```python
from build123d import *

# Parameters (mm, degrees)
SKETCH1_R           = 2.5527
SKETCH1_R_2         = 19.685
SKETCH1_W           = 12.7
SKETCH1_H           = 12.7
BOSS_EXTRUDE1_DEPTH = 14.605
CUT_EXTRUDE1_DEPTH  = 6.35
BOSS_EXTRUDE2_START = -5.842
SKETCH3_R           = 19.685
SKETCH3_R_2         = 14.2875
BOSS_EXTRUDE2_DEPTH = 5.842
SKETCH4_R           = 2.5527
CUT_EXTRUDE2_DEPTH  = 93.738266239
CUT_EXTRUDE3_DEPTH  = 6.35
CUT_EXTRUDE4_START  = -7.62
SKETCH8_R           = 2.5527
CUT_EXTRUDE4_DEPTH  = 7.62
FILLET1_R           = 3.81
FILLET3_R           = 0.0635
FILLET4_START       = 6.985
FILLET4_DEPTH       = 9.015
CHAMFER1_SIZE       = 3.81
FILLET5_R           = 2.54


with BuildPart() as part:
    # Sketch1 → Boss-Extrude1 (new body)
    # profile 1 of 3: a face of its own
    with BuildSketch(Plane.XY):
        Polygon((0, 63.5), (0, 0), (50.8, 0), (50.8, 63.5), (38.1, 63.5), (12.7, 63.5), align=None)
        with Locations(Location((6.35, 6.35, 0), (0, 0, 180))):
            Circle(SKETCH1_R, mode=Mode.SUBTRACT)
        with Locations(Location((5.668864874, 22.104928677, 0), (0, 0, 180))):
            Circle(SKETCH1_R, mode=Mode.SUBTRACT)
        with Locations(Location((44.45, 6.35, 0), (0, 0, 180))):
            Circle(SKETCH1_R, mode=Mode.SUBTRACT)
        with Locations(Location((44.45, 19.05, 0), (0, 0, 180))):
            Circle(SKETCH1_R, mode=Mode.SUBTRACT)
        with Locations(Location((25.4, 38.1, 0), (0, 0, 180))):
            Circle(SKETCH1_R_2, mode=Mode.SUBTRACT)
        with Locations(Location((45.131135126, 54.095071323, 0), (0, 0, 180))):
            Circle(SKETCH1_R, mode=Mode.SUBTRACT)
    # profile 2 of 3: a face of its own
    with BuildSketch(Plane.XY):
        with Locations((6.35, 69.85)):
            Rectangle(SKETCH1_W, SKETCH1_H)
        with Locations(Location((6.35, 69.85, 0), (0, 0, 180))):
            Circle(SKETCH1_R, mode=Mode.SUBTRACT)
    # profile 3 of 3: a face of its own
    with BuildSketch(Plane.XY):
        with Locations((44.45, 69.85)):
            Rectangle(SKETCH1_W, SKETCH1_H)
        with Locations(Location((44.45, 67.945, 0), (0, 0, 180))):
            Circle(SKETCH1_R, mode=Mode.SUBTRACT)
    extrude(amount=BOSS_EXTRUDE1_DEPTH)

    # Sketch2 → Cut-Extrude1 (cut)
    with BuildSketch(Plane(origin=(0, 0, 0), x_dir=(-1, 0, 0), z_dir=(0, 0, -1))):
        Polygon((-41.45488381, 58.476257037), (-47.087227595, 59.469391211), (-50.763478911, 55.088205497), (-48.807386443, 49.713885609), (-43.175042658, 48.720751435), (-39.498791341, 53.101937149), align=None)
        Polygon((-1.992613557, 26.486114391), (-7.624957342, 27.479248565), (-11.301208659, 23.098062851), (-9.34511619, 17.723742963), (-3.712772405, 16.730608789), (-0.036521089, 21.111794503), align=None)
        Polygon((-41.590384117, 11.303), (-47.309615883, 11.303), (-50.169231767, 6.35), (-47.309615883, 1.397), (-41.590384117, 1.397), (-38.730768233, 6.35), align=None)
        Polygon((-44.45, 73.664231767), (-49.403, 70.804615883), (-49.403, 65.085384117), (-44.45, 62.225768233), (-39.497, 65.085384117), (-39.497, 70.804615883), align=None)
    extrude(amount=-CUT_EXTRUDE1_DEPTH, mode=Mode.SUBTRACT)

    # Sketch3 → Boss-Extrude2 (add)
    with BuildSketch(Plane.XY.offset(14.605).offset(BOSS_EXTRUDE2_START)):
        with Locations(Location((25.4, 38.1, 0), (0, 0, 180))):
            Circle(SKETCH3_R)
        with Locations((25.4, 38.1)):
            Circle(SKETCH3_R_2, mode=Mode.SUBTRACT)
    extrude(amount=BOSS_EXTRUDE2_DEPTH)

    # Sketch4 → Cut-Extrude2 (cut, through all)
    with BuildSketch(Plane.XY.offset(14.605)):
        with Locations((6.35, 54.61)):
            Circle(SKETCH4_R)
    extrude(amount=-CUT_EXTRUDE2_DEPTH, mode=Mode.SUBTRACT)

    # Sketch5 → Cut-Extrude3 (cut)
    with BuildSketch(Plane(origin=(0, 0, 0), x_dir=(-1, 0, 0), z_dir=(0, 0, -1))):
        Polygon((-2.673748684, 50.228814286), (-0.717656215, 55.603134174), (-4.393907531, 59.984319888), (-10.026251316, 58.991185714), (-11.982343785, 53.616865826), (-8.306092469, 49.235680112), align=None)
    extrude(amount=-CUT_EXTRUDE3_DEPTH, mode=Mode.SUBTRACT)

    # Sketch8 → Cut-Extrude4 (cut)
    # profile 1 of 3: a face of its own
    with BuildSketch(Plane.XY.offset(14.605).offset(CUT_EXTRUDE4_START)):
        with BuildLine():
            Line((0, 76.2), (0, 69.85))
            ThreePointArc((0, 69.85), (6.35, 63.5), (12.7, 69.85))
            Line((12.7, 69.85), (12.7, 76.2))
            Line((12.7, 76.2), (0, 76.2))
        make_face()
        with Locations(Location((6.35, 69.85, 0), (0, 0, 180))):
            Circle(SKETCH8_R, mode=Mode.SUBTRACT)
    # profile 2 of 3: a face of its own
    with BuildSketch(Plane.XY.offset(14.605).offset(CUT_EXTRUDE4_START)):
        with BuildLine():
            Line((50.8, 25.4), (44.45, 25.4))
            ThreePointArc((44.45, 25.4), (38.1, 19.05), (44.45, 12.7))
            Line((44.45, 12.7), (50.8, 12.7))
            Line((50.8, 12.7), (50.8, 25.4))
        make_face()
        with Locations(Location((44.45, 19.05, 0), (0, 0, 180))):
            Circle(SKETCH8_R, mode=Mode.SUBTRACT)
    # profile 3 of 3: a face of its own
    with BuildSketch(Plane.XY.offset(14.605).offset(CUT_EXTRUDE4_START)):
        with BuildLine():
            Line((0, 0), (6.35, 0))
            ThreePointArc((6.35, 0), (10.840128061, 10.840128061), (0, 6.35))
            Line((0, 6.35), (0, 0))
        make_face()
        with Locations(Location((6.35, 6.35, 0), (0, 0, 180))):
            Circle(SKETCH8_R, mode=Mode.SUBTRACT)
    extrude(amount=CUT_EXTRUDE4_DEPTH, mode=Mode.SUBTRACT)

    # Fillet1
    fillet1_edges = [part.edges().sort_by_distance(p)[0] for p in [
        (0, 0, 3.4925),
        (0, 76.2, 3.4925),
        (12.7, 76.2, 3.4925),
        (12.7, 63.5, 7.3025),
        (38.1, 63.5, 7.3025),
        (38.1, 76.2, 7.3025),
        (50.8, 76.2, 7.3025),
        (50.8, 0, 7.3025),
    ]]
    fillet(fillet1_edges, radius=FILLET1_R)

    # Fillet3
    fillet3_edges = [part.edges().sort_by_distance(p)[0] for p in [
        (45.085, 38.1, 8.763),
    ]]
    fillet(fillet3_edges, radius=FILLET3_R)

    # Fillet4: read off the stored shape, not the designer's step
    # Fillet4 outline → Fillet4 (cut)
    with BuildSketch(Plane.XY.offset(FILLET4_START)):
        with BuildLine():
            ThreePointArc((14.382185257, 0), (12.23549345, 1.182312891), (12.087275183, 3.628571429))
            ThreePointArc((12.087275183, 3.628571429), (9.744217773, 0.983270482), (6.35, 0))
            Line((6.35, 0), (14.382185257, 0))
        make_face()
        with BuildLine():
            ThreePointArc((3.628571429, 12.087275183), (1.182312891, 12.23549345), (0, 14.382185257))
            Line((0, 14.382185257), (0, 6.35))
            ThreePointArc((0, 6.35), (0.983270482, 9.744217773), (3.628571429, 12.087275183))
        make_face()
        with BuildLine():
            ThreePointArc((0, 61.817814743), (1.182312891, 63.96450655), (3.628571429, 64.112724817))
            ThreePointArc((3.628571429, 64.112724817), (0.983270483, 66.455782228), (0, 69.85))
            Line((0, 69.85), (0, 61.817814743))
        make_face()
        with BuildLine():
            ThreePointArc((12.7, 69.85), (12.076615103, 67.106210748), (10.328856864, 64.901141742))
            ThreePointArc((10.328856864, 64.901141742), (12.086184936, 65.456182276), (13.756239766, 64.676959064))
            ThreePointArc((13.756239766, 64.676959064), (12.973905651, 65.891501938), (12.7, 67.31))
            Line((12.7, 67.31), (12.7, 69.85))
        make_face()
    extrude(amount=FILLET4_DEPTH, mode=Mode.SUBTRACT)

    # Chamfer1
    # the kernel refuses this chamfer: 3.81 mm, written as the material it takes off along each edge
    with BuildSketch(Plane(origin=(60.598112184, 25.4, 14.605), x_dir=(0, 1, 0), z_dir=(-1, 0, 0)), Plane(origin=(44.45, 12.7, 14.605), x_dir=(0, -1, 0), z_dir=(1, 0, 0))) as chamfer1_piece_1:
        Polygon((CHAMFER1_SIZE, 0), (0, CHAMFER1_SIZE), (0, 0), align=None)
    extrude(amount=16.148112184, mode=Mode.SUBTRACT)
    with BuildSketch(Plane(origin=(44.45, 19.05, 14.605), x_dir=(0, 1, 0), z_dir=(1, 0, 0))) as chamfer1_piece_2:
        Polygon((6.35 + CHAMFER1_SIZE, 0), (6.35, -CHAMFER1_SIZE), (6.35, 0), align=None)
    revolve(axis=Axis((44.45, 19.05, 14.605), (0, 0, 1)), revolution_arc=180, mode=Mode.SUBTRACT)

    # Fillet5
    fillet5_edges = [part.edges().sort_by_distance(p)[0] for p in [
        (25.4, 63.5, 14.605),
        (50.8, 6.35, 14.605),
        (44.45, 76.2, 14.605),
        (38.1, 69.85, 14.605),
        (39.215923164, 75.084076836, 14.605),
        (49.684076836, 75.084076836, 14.605),
        (49.684076836, 1.115923164, 14.605),
        (15.012633306, 63.806574108, 14.605),
        (36.984076836, 64.615923164, 14.605),
        (7.092079369, 63.543509834, 14.605),
        (30.686092628, 0, 14.605),
        (0, 38.1, 14.605),
        (10.840128061, 10.840128061, 14.605),
        (1.182312891, 12.23549345, 14.605),
        (12.23549345, 1.182312891, 14.605),
        (12.086184936, 65.456182276, 14.605),
        (1.182312891, 63.96450655, 14.605),
        (50.8, 50.8, 14.605),
    ]]
    fillet(fillet5_edges, radius=FILLET5_R)


solid = part.part
```
Model file for the job. Use its own axes, mm. A direction names the side the tool comes from. Coordinates: 2 decimals unless noted, no trailing zeros. Answer as a JSON object with one key per item and string values. Group by question number.
(1) Flat gauge pins, fed straight in: pin 1 (8 mm diameter, centred on x = 21.5, y = 67, fed in from +Z); pin 2 (6 mm diameter, centred on x = 20.5, z = 4, fed in from +Y); pin 3 (7 mm diameter, centred on x = 4, y = 5.5, fed in from +Z) (3 decimals). Where does each tip first touch, or does it go through?
(2) Cut at B-B (z = 5.5). State how many separate pieces and enclosed holes the cut face has, then the cut area to 3 significant figures.
(3) Tool access for faces 1 (the face through (43, 9, 6.35)), 2 (the face through (48, 25.4, 9)), 3 (the face through (12.7, 70, 3)): list every direction of +Z, -Z, +X, -X, +Y, -Y with a clear straight run to the whole face (end or side of a thin tool).
(4) Probe line 1 along Y through (x, z) = (25.4, 5.25) (3 decimals); line 2 along X through (y, z) = (69, 6.25); line 3 along Y through (x, z) = (43, 5.25). List the from-to ranges inside material, lowest first.
(5) Two-plate mould, pull along X, no slides. Class faces 4 (the face through (47, 67, 6.35)), 5 (the face through (44, 11.303, 3)), 6 (the face through (12.255, 1.152, 9.489)), 7 (the face through (48, 12.7, 9)): released by +X, released by -X, zero draft, split by the parting line, or undercut.
Geometry says:
{
 "1": {"pin 1": "stops at z = 13.58", "pin 2": "stops at y = 63.5", "pin 3": "stops at z = 6.985"},
 "2": {"separate pieces": "1", "enclosed holes": "9", "area": "1,830 mm^2"},
 "3": {"face 1": "-Z", "face 2": "+Z, +X", "face 3": "+Z, -Z, +Y"},
 "4": {"line 1": "y = 0 to 18.415, 57.785 to 63.5", "line 2": "x = 0 to 3.94, 8.76 to 12.7, 38.1 to 39.5, 49.4 to 50.8", "line 3": "y = 0 to 1.4, 11.3 to 16.95, 21.15 to 29.28, 46.92 to 48.93, 58.75 to 63.06, 72.83 to 76.2"},
 "5": {"face 4": "undercut", "face 5": "undercut", "face 6": "released by -X", "face 7": "zero draft"}
}
